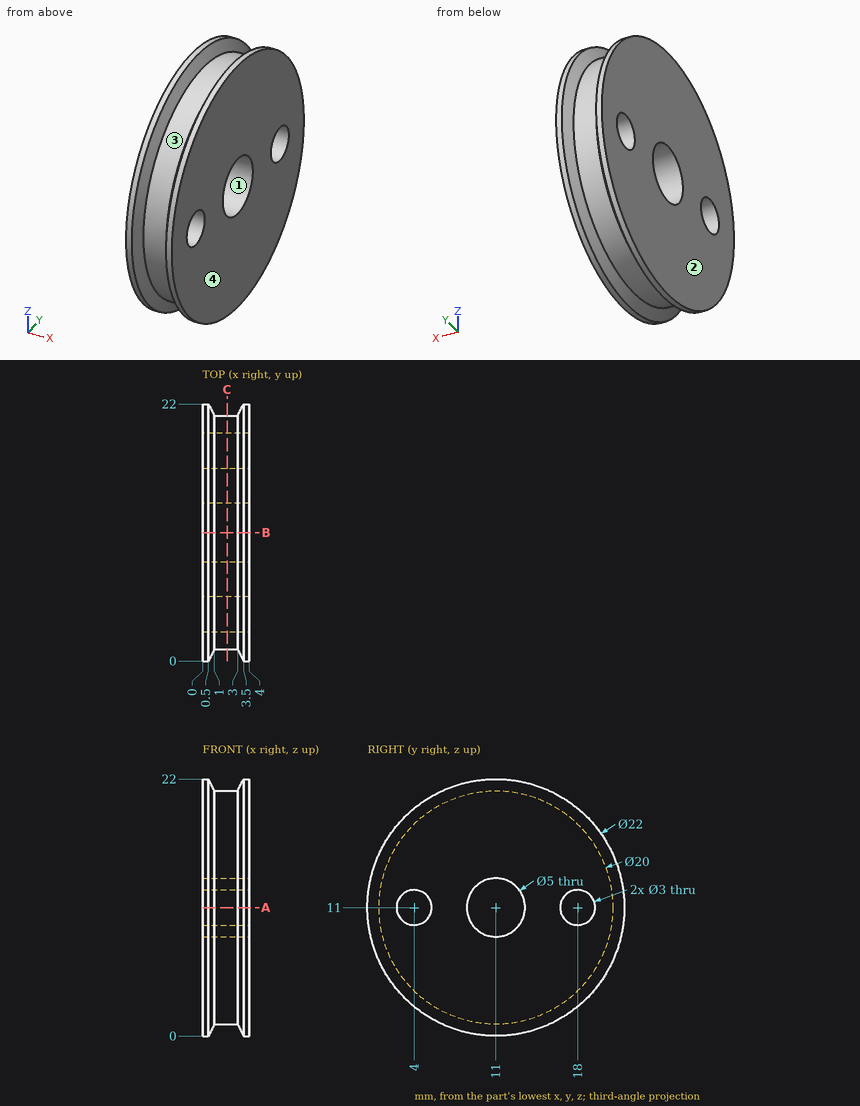
Geometry: see drawing. Coordinates: mm, zero at the bounding-box minimum. Round coordinates to 2 decimals unless told otherwise and drop trailing zeros. Loops run counter-clockwise (first coordinate to the right, second up) from the corner with the lowest first, then second, coordinate; pieces in that order, holes last. Notation, with made-up numbers: M -5,46.5 L 23,46.5 A7 cw 23,50.5 Z; hole C 10.25,45.25 d3. An arc over 180 degrees is marked long. Use a Markdown table: item, result. Add a question column.
1. Cut plane A-A, the plane z = 11. Output: boundary loops of the cut face in (x, y).
2. Ray query, line 1 along Z through (x, y) = (2.75, 4); line 2 along Z through (x, y) = (0.55, 11); line 3 along Y through (x, z) = (2.4, 8). Return the intervals inside material, ascending. Write a range as [from, to].
3. Pull-direction query (X, two-part tool) for the marked faces 1, 2, 3 and 4; classes: +X half, -X half, draft (parallel to the pull), parting line (faces both ways), or undercut.
4. Contact query for a flat-ended pin moving along its axis: pin 1 (1.5 mm diameter, centred on x = 3, y = 3.5, fed in from +Z). Output: stop coordinate, or through.
5. Cut plane C-C, the plane x = 2.1. Output: boundary loops of the cut face in (y, z), and give its area (3 significant figures).
6. Cut plane B-B, the plane y = 11. Output: boundary loops of the cut face in (x, z), and give its area (3 significant figures).
Solution:
| question | item | result |
|---|---|---|
| 1 | outline | M 0,0 L 0.5,0 L 1,1 L 3,1 L 3.5,0 L 4,0 L 4,2.5 L 0,2.5 Z; M 0,5.5 L 4,5.5 L 4,8.5 L 0,8.5 Z; M 0,13.5 L 4,13.5 L 4,16.5 L 0,16.5 Z; M 0,19.5 L 4,19.5 L 4,22 L 3.5,22 L 3,21 L 1,21 L 0.5,22 L 0,22 Z |
| 2 | line 1 | z = [3.86, 9.5], [12.5, 18.14] |
| 2 | line 2 | z = [0.1, 8.5], [13.5, 21.9] |
| 2 | line 3 | y = [1.46, 20.54] |
| 3 | face 1 | draft |
| 3 | face 2 | -X half |
| 3 | face 3 | undercut |
| 3 | face 4 | +X half |
| 4 | pin 1 | stops at z = 19.53 |
| 5 | outline | C 11,11 d20; hole C 4,11 d3; hole C 11,11 d5; hole C 18,11 d3 |
| 5 | area | 280 mm2 |
| 6 | outline | M 0,0 L 0.5,0 L 1,1 L 3,1 L 3.5,0 L 4,0 L 4,8.5 L 0,8.5 Z; M 0,13.5 L 4,13.5 L 4,22 L 3.5,22 L 3,21 L 1,21 L 0.5,22 L 0,22 Z |
| 6 | area | 63.0 mm2 |
